from build123d import *

# Parameters (mm, degrees)
SKETCH1_W                  = 25.4
SKETCH1_H                  = 1498.6
BOSS_EXTRUDE1_DEPTH        = 25.4
SKETCH2_W                  = 23.114
SKETCH2_H                  = 23.114
CUT_EXTRUDE1_DEPTH         = 1499.6
M3_5_CLEARANCE_HOLE1_D     = 4.1402
M3_5_CLEARANCE_HOLE1_DEPTH = 25.4
M3_5_CLEARANCE_HOLE2_D     = 4.1402
M3_5_CLEARANCE_HOLE2_DEPTH = 25.4
CHAMFER1_SIZE              = 2.159
FILLET1_R                  = 0.8128
FILLET2_R                  = 3.0988
SKETCH8_W                  = 95.882963774
SKETCH8_H                  = 79.338329604
CUT_EXTRUDE3_DEPTH         = 1371.6
SKETCH11_W                 = 51.462522779
SKETCH11_H                 = 66.676735099
CUT_EXTRUDE6_DEPTH         = 2.286
SKETCH12_W                 = 22.3012
SKETCH12_H                 = 61.214
CUT_EXTRUDE7_DEPTH         = 2.54


with BuildPart() as part:
    # Sketch1 → Boss-Extrude1 (new body)
    with BuildSketch(Plane(origin=(0, 0, 0), x_dir=(0, -1, 0), z_dir=(-1, 0, 0))):
        with Locations((-12.7, 0)):
            Rectangle(SKETCH1_W, SKETCH1_H)
    extrude(amount=-BOSS_EXTRUDE1_DEPTH)

    # Sketch2 → Cut-Extrude1 (cut, through all)
    with BuildSketch(Plane(origin=(0, 0, -749.3), x_dir=(-1, 0, 0), z_dir=(0, 0, -1))):
        with Locations((-13.843, 13.843)):
            Rectangle(SKETCH2_W, SKETCH2_H)
    extrude(amount=-CUT_EXTRUDE1_DEPTH, mode=Mode.SUBTRACT)

    # M3.5 Clearance Hole1
    with Locations(Plane(origin=(0, 0, 0), x_dir=(-1, 0, 0), z_dir=(0, -1, 0))):
        with Locations((-12.7, 736.6), (-12.7, 711.2), (-12.7, 685.8), (-12.7, 660.4), (-12.7, 635), (-12.7, 609.6), (-12.7, 584.2), (-12.7, 558.8), (-12.7, 533.4), (-12.7, 508), (-12.7, 482.6), (-12.7, 457.2), (-12.7, 431.8), (-12.7, 406.4), (-12.7, 381), (-12.7, 355.6), (-12.7, 330.2), (-12.7, 304.8), (-12.7, 279.4), (-12.7, 254), (-12.7, 228.6), (-12.7, 203.2), (-12.7, 177.8), (-12.7, 152.4), (-12.7, 127), (-12.7, 101.6), (-12.7, 76.2), (-12.7, 50.8), (-12.7, 25.4), (-12.7, 0), (-12.7, -25.4), (-12.7, -50.8), (-12.7, -76.2), (-12.7, -101.6), (-12.7, -127), (-12.7, -152.4), (-12.7, -177.8), (-12.7, -203.2), (-12.7, -228.6), (-12.7, -254), (-12.7, -279.4), (-12.7, -304.8), (-12.7, -330.2), (-12.7, -355.6), (-12.7, -381), (-12.7, -406.4), (-12.7, -431.8), (-12.7, -457.2), (-12.7, -482.6), (-12.7, -508), (-12.7, -533.4), (-12.7, -558.8), (-12.7, -584.2), (-12.7, -609.6), (-12.7, -635), (-12.7, -660.4), (-12.7, -685.8), (-12.7, -711.2), (-12.7, -736.6)):
            Hole(M3_5_CLEARANCE_HOLE1_D / 2, depth=M3_5_CLEARANCE_HOLE1_DEPTH)

    # M3.5 Clearance Hole2
    with Locations(Plane.ZY):
        with Locations((711.2, 12.7), (736.6, 12.7), (685.8, 12.7), (660.4, 12.7), (635, 12.7), (609.6, 12.7), (584.2, 12.7), (558.8, 12.7), (533.4, 12.7), (508, 12.7), (482.6, 12.7), (457.2, 12.7), (431.8, 12.7), (406.4, 12.7), (381, 12.7), (355.6, 12.7), (330.2, 12.7), (304.8, 12.7), (279.4, 12.7), (254, 12.7), (228.6, 12.7), (203.2, 12.7), (177.8, 12.7), (152.4, 12.7), (127, 12.7), (101.6, 12.7), (76.2, 12.7), (50.8, 12.7), (25.4, 12.7), (0, 12.7), (-25.4, 12.7), (-50.8, 12.7), (-76.2, 12.7), (-101.6, 12.7), (-127, 12.7), (-152.4, 12.7), (-177.8, 12.7), (-203.2, 12.7), (-228.6, 12.7), (-254, 12.7), (-279.4, 12.7), (-304.8, 12.7), (-330.2, 12.7), (-355.6, 12.7), (-381, 12.7), (-406.4, 12.7), (-431.8, 12.7), (-457.2, 12.7), (-482.6, 12.7), (-508, 12.7), (-533.4, 12.7), (-558.8, 12.7), (-584.2, 12.7), (-609.6, 12.7), (-635, 12.7), (-660.4, 12.7), (-685.8, 12.7), (-711.2, 12.7), (-736.6, 12.7)):
            Hole(M3_5_CLEARANCE_HOLE2_D / 2, depth=M3_5_CLEARANCE_HOLE2_DEPTH)

    # Chamfer1
    chamfer1_edges = [part.edges().sort_by_distance(p)[0] for p in [
        (25.4, 1.143, -749.3),
        (1.143, 25.4, 749.3),
        (1.143, 25.4, -749.3),
        (25.4, 1.143, 749.3),
    ]]
    chamfer(chamfer1_edges, length=CHAMFER1_SIZE)

    # Fillet1
    fillet1_edges = [part.edges().sort_by_distance(p)[0] for p in [
        (2.286, 2.286, 0),
    ]]
    fillet(fillet1_edges, radius=FILLET1_R)

    # Fillet2
    fillet2_edges = [part.edges().sort_by_distance(p)[0] for p in [
        (0, 0, 0),
    ]]
    fillet(fillet2_edges, radius=FILLET2_R)

    # Sketch8 → Cut-Extrude3 (cut)
    with BuildSketch(Plane.XY.offset(749.3)):
        with Locations((2.286, 3.0988)):
            Rectangle(SKETCH8_W, SKETCH8_H)
    extrude(amount=-CUT_EXTRUDE3_DEPTH, mode=Mode.SUBTRACT)

    # Sketch11 → Cut-Extrude6 (cut)
    with BuildSketch(Plane.XY.offset(-622.3)):
        with Locations((1.85517497, 1.74884985)):
            Rectangle(SKETCH11_W, SKETCH11_H)
    extrude(amount=-CUT_EXTRUDE6_DEPTH, mode=Mode.SUBTRACT)

    # Sketch12 → Cut-Extrude7 (cut)
    with BuildSketch(Plane(origin=(0, 2.286, 0), x_dir=(1, 0, 0), z_dir=(0, 1, 0))):
        with Locations((14.2494, 655.193)):
            Rectangle(SKETCH12_W, SKETCH12_H)
    extrude(amount=-CUT_EXTRUDE7_DEPTH, mode=Mode.SUBTRACT)


solid = part.part
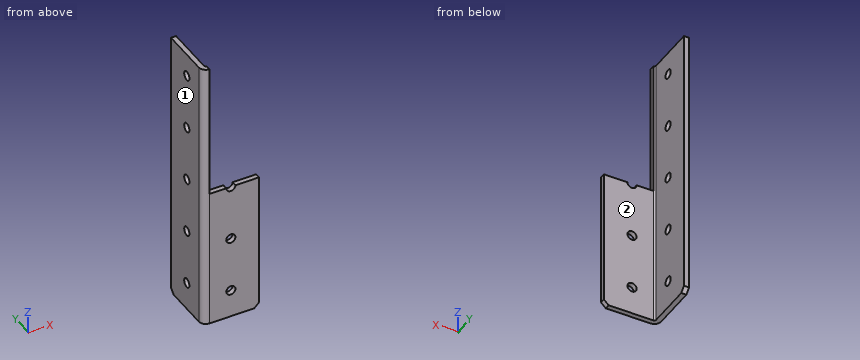
Work out the finished part from the listing and answer in its coordinate system (mm). Face numbers are marked on the shaded views. A direction names the side the tool comes from. Give positions to 0.01 mm unless a question says otherwise; leave off trailing zeros. Write each loop counter-clockwise with the first axis right and the second up, starting at its lowest first coordinate (ties: lowest second). Pieces come first, ordered by that corner, then holes. Notation, with made-up numbers: M -23,65 L -7,65 A18 cw -7,74 Z; hole C -10,-23.75 d6. An arc over 180 degrees is marked long. Answer as CSV lines item,"result".
Q1. A cutting plane is placed at D-D on z = -711.2. Write down the section's boundary in (x, y).
A:
outline,"M 0,3.1 A3.1 ccw 3.1,0 L 10.63,0 L 10.63,2.29 L 3.1,2.29 A0.81 cw 2.29,3.1 L 2.29,10.63 L 0,10.63 Z; M 0,14.77 L 2.29,14.77 L 2.29,25.4 L 0,25.4 Z; M 14.77,0 L 25.4,0 L 25.4,2.29 L 14.77,2.29 Z"
Q2. A cutting plane is placed at C-C on y = 12.7. Write down the section's boundary in (x, z).
A:
outline,"M 0,-749.3 L 2.29,-749.3 L 2.29,-738.67 L 0,-738.67 Z; M 0,-734.53 L 2.29,-734.53 L 2.29,-713.27 L 0,-713.27 Z; M 0,-709.13 L 2.29,-709.13 L 2.29,-687.87 L 0,-687.87 Z; M 0,-683.73 L 2.29,-683.73 L 2.29,-662.47 L 0,-662.47 Z; M 0,-658.33 L 2.29,-658.33 L 2.29,-637.07 L 0,-637.07 Z; M 0,-632.93 L 2.29,-632.93 L 2.29,-624.59 L 0,-624.59 Z"
Q3. A cutting plane is placed at B-B on x = 12.7. Write down the section's boundary in (y, z), plus the area to 4 significant figures.
A:
outline,"M 0,-749.3 L 2.29,-749.3 L 2.29,-738.67 L 0,-738.67 Z; M 0,-734.53 L 2.29,-734.53 L 2.29,-713.27 L 0,-713.27 Z; M 0,-709.13 L 2.29,-709.13 L 2.29,-687.87 L 0,-687.87 Z"
area,"121.5 mm²"
Q4. A cutting plane is placed at A-A on z = -660.4. Write down the section's boundary in (x, y).
A:
outline,"M 0,3.1 A3.1 ccw 3.1,0 L 3.1,2.29 A0.81 cw 2.29,3.1 L 2.29,10.63 L 0,10.63 Z; M 0,14.77 L 2.29,14.77 L 2.29,25.4 L 0,25.4 Z"
Q5. A tool of negligible diameter and unlimited length cuts with its end or side. For the marked faces 1 and 2, from which of +Z, -Z, +X, -X, +Y, -Y can it reach the whole face along a straight path? Write none if from no direction.
A:
face 1,"+Z, -Z, -X, +Y, -Y"
face 2,"+Z, -Z, +X, +Y"
Q6. Find the intervals of material crossed by probe 1 along Z at (x, y) = (12.7, 1.75); probe 2 along X at (y, z) = (18.5, -647); probe 3 along Y at (x, z) = (1.75, -736.6), in increasing order. Write a range as [from, to].
A:
probe 1,"z = [-749.3, -738.67], [-734.53, -713.27], [-709.13, -687.87]"
probe 2,"x = [0, 2.29]"
probe 3,"y = [0.31, 10.63], [14.77, 25.4]"
Q7. Given P1, Ø1.1, axis at x = 19, y = 1.5, coming from the +Z side; P2, Ø2, axis at y = 8, z = -654.5, coming from the +X side; P3, Ø6.5, axis at x = 12.7, z = -736.6, coming from the +Y side; P4, Ø4, axis at x = 18.5, y = 4.5, coming from the +Z side, each flat-ended and moving along its own axis, determine where each tip first touches the part or whether it passes through.
A:
P1,"stops at z = -685.8"
P2,"stops at x = 2.29"
P3,"stops at y = 2.29"
P4,"passes through"
